Here's the drawing with two shaded views (mm, measured from the low corner). I have some questions. A direction names the side the tool comes from. Coordinates: 2 decimals unless noted, no trailing zeros. Order: outer loops, then holes, each group sorted by start corner. A loop starts at its lowest first (then second) coordinate and runs counter-clockwise, first axis right, second up. Notation, with made-up numbers: M -12,36 L 22,36 A17 cw 22,45 Z; hole C -14.75,-24.75 d10. An arc over 180 degrees is marked long. Put each result on its own line as item: value. Start each with the question number.
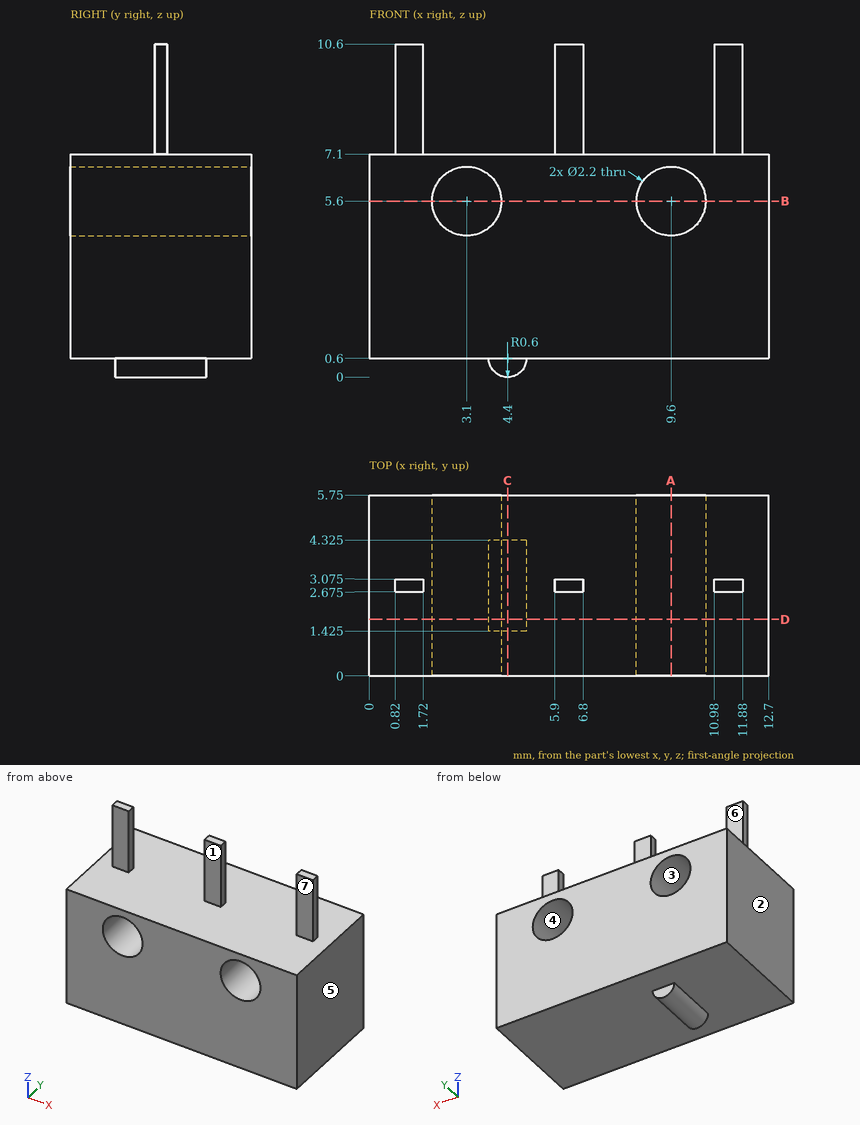
Item 1: For the marked faces 5, 6 and 7, which set-ups out of +Z, -Z, +X, -X, +Y, -Y let a thin tool reach every point of the face, with its end or its side?
Item 2: For pin 1 Ø0.5 at (x, z) = (11.5, 9) entering from +Y (3 decimals); pin 2 Ø1.5 at (y, z) = (3.5, 9) entering from +X; pin 3 Ø0.5 at (x, z) = (6.5, 9.5) entering from -Y (3 decimals), each with a flat end and sliding along its axis, tell me the tip position at first contact or that it passes through.
Item 3: If we section it at B-B on z = 5.6: Write out the boundary of the cut face in (x, y), then the cut area to 3 significant figures.
Item 4: If we mould it in two halves opening along X, with no side actions, what happens to the marked faces 1, 2, 3 and 4? For each: released by +X, released by -X, zero draft, split by the parting line, or undercut.
Item 5: If we section it at A-A on x = 9.6: Write out the boundary of the cut face in (y, z), then the cut area to 3 significant figures.
Item 6: I need wall thicknesses on probe 1 along X at (y, z) = (1.55, 5.6); probe 2 along Z at (x, y) = (9.6, 2.8); probe 3 along Y at (x, z) = (11.75, 9.25) (3 decimals). Which ranges of each line are inside material? Lowest first, please.
Item 7: If we section it at C-C on x = 4.4: Write out the boundary of the cut face in (y, z) (3 decimals), then the cut area to 3 significant figures.
Item 8: If we section it at D-D on y = 1.8: Write out the boundary of the cut face in (x, z).
Geometry check:
1. face 5: +Z, -Z, +X, +Y, -Y
1. face 6: +Z, +X, -X, +Y
1. face 7: +Z, +X, -X, -Y
2. pin 1: stops at y = 3.075
2. pin 2: stops at x = 11.88
2. pin 3: stops at y = 2.675
3. outline: M 0,0 L 2,0 L 2,5.75 L 0,5.75 Z; M 4.2,0 L 8.5,0 L 8.5,5.75 L 4.2,5.75 Z; M 10.7,0 L 12.7,0 L 12.7,5.75 L 10.7,5.75 Z
3. area: 47.7 mm²
4. face 1: zero draft
4. face 2: released by -X
4. face 3: undercut
4. face 4: undercut
5. outline: M 0,0.6 L 5.75,0.6 L 5.75,4.5 L 0,4.5 Z; M 0,6.7 L 5.75,6.7 L 5.75,7.1 L 0,7.1 Z
5. area: 24.7 mm²
6. probe 1: x = 0 to 2, 4.2 to 8.5, 10.7 to 12.7
6. probe 2: z = 0.6 to 4.5, 6.7 to 7.1
6. probe 3: y = 2.675 to 3.075
7. outline: M 0,0.6 L 1.425,0.6 L 1.425,0 L 4.325,0 L 4.325,0.6 L 5.75,0.6 L 5.75,7.1 L 0,7.1 Z
7. area: 39.1 mm²
8. outline: M 0,0.6 L 3.8,0.6 A0.6 ccw 5,0.6 L 12.7,0.6 L 12.7,7.1 L 0,7.1 Z; hole C 3.1,5.6 d2.2; hole C 9.6,5.6 d2.2
